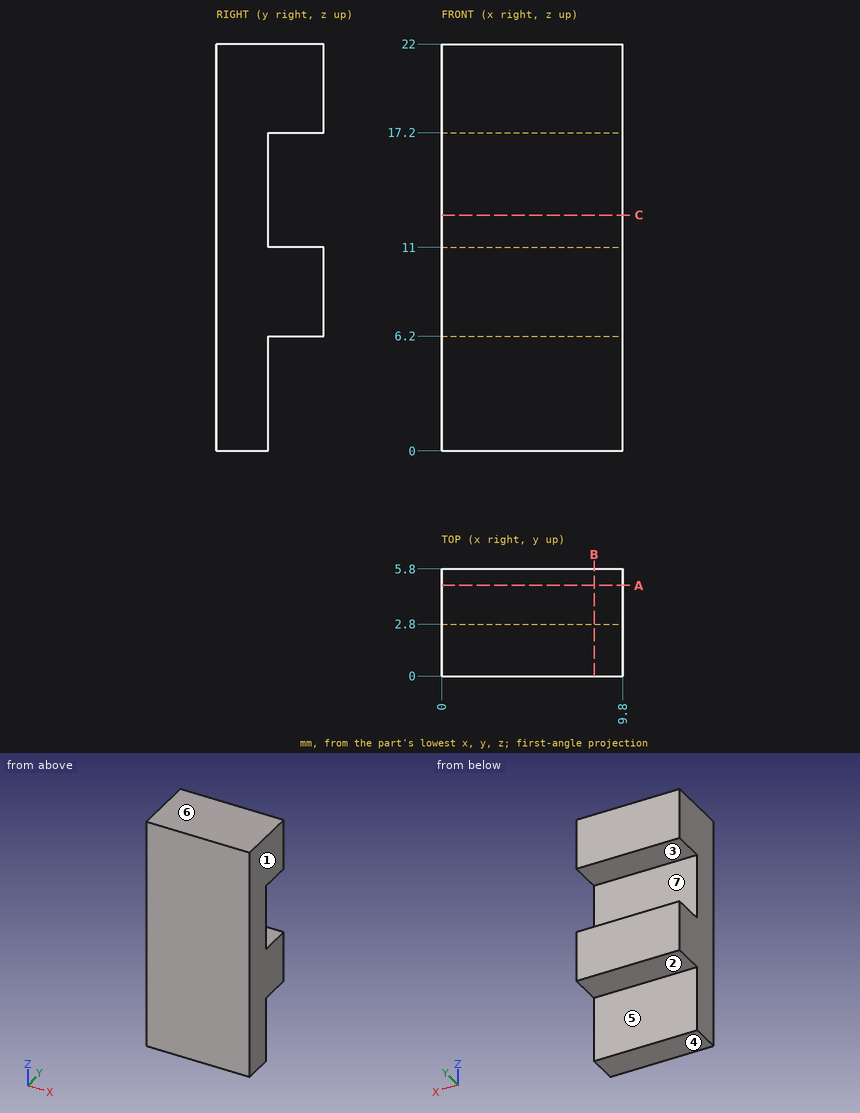
Geometry check sheet. Reference: drawing and pictorial views, mm from the part's lowest x, y, z. A direction names the side the tool comes from. Round coordinates to 2 decimals unless told otherwise and drop trailing zeros. Order: outer loops, then holes, each group sorted by start corner. A loop starts at its lowest first (then second) coordinate and runs counter-clockwise, first axis right, second up. Notation, with made-up numbers: (70, 63) - (119, 63) arc R20 cw to (119, 86) - close; hole circle Ø9 at (89, -24.75). An arc over 180 degrees is marked (long way). Use a Markdown table: item, result. Add a question column.
1) Mould release check, pull along Z, two halves, no side actions. Record for the marked faces 4, 5, 6 and 7: released by +Z, released by -Z, zero draft, split by the parting line, or undercut.
2) Section check C-C (z = 12.75). Record the cut outline in (x, y).
3) Section check A-A (y = 4.9). Record the cut outline in (x, z).
4) Set-up check for the marked faces 1, 2 and 3: record each of +Z, -Z, +X, -X, +Y, -Y from which the full face is reachable in a straight line by a thin tool's end or side.
5) Section check B-B (x = 8.25). Record the cut outline in (y, z), then the cut area to 3 significant figures.
6) Thickness scan on line 1 along Z through (x, y) = (1.25, 3.45); line 2 along Y through (x, z) = (7.5, 6). Record the ranges inside material, lowest first.
7) Gauge pin test, flat ends, axial feed: P1, Ø5, axis at x = 6.5, z = 3.5, coming from the +Y side; P2, Ø0.9, axis at x = 4.5, y = 5, coming from the -Z side. Record the tip position at first contact, or that the pin passes through.
Established:
| question | item | result |
|---|---|---|
| 1 | face 4 | released by -Z |
| 1 | face 5 | zero draft |
| 1 | face 6 | released by +Z |
| 1 | face 7 | undercut |
| 2 | outline | (0, 0) - (9.8, 0) - (9.8, 2.8) - (0, 2.8) - close |
| 3 | outline | (0, 6.2) - (9.8, 6.2) - (9.8, 11) - (0, 11) - close; (0, 17.2) - (9.8, 17.2) - (9.8, 22) - (0, 22) - close |
| 4 | face 1 | +Z, -Z, +X, +Y, -Y |
| 4 | face 2 | -Z, +X, -X, +Y |
| 4 | face 3 | +X, -X, +Y |
| 5 | outline | (0, 0) - (2.8, 0) - (2.8, 6.2) - (5.8, 6.2) - (5.8, 11) - (2.8, 11) - (2.8, 17.2) - (5.8, 17.2) - (5.8, 22) - (0, 22) - close |
| 5 | area | 90.4 mm2 |
| 6 | line 1 | 6.2 to 11, 17.2 to 22 |
| 6 | line 2 | 0 to 2.8 |
| 7 | P1 | y = 2.8 |
| 7 | P2 | z = 6.2 |
